```python
from build123d import *

# Parameters (mm, degrees)
SKETCH025_R     = 152.5
PAD015_DEPTH    = 8
SKETCH057_R     = 145.5
PAD016_DEPTH    = 4
SKETCH052_R     = 3
SKETCH052_R_2   = 1.5
SKETCH052_R_3   = 1
SKETCH052_R_4   = 2.75
POCKET018_DEPTH = 12.001


with BuildPart() as part:
    # Sketch025 → Pad015 (new body)
    with BuildSketch(Plane.XY):
        with Locations((0.142028, -323.737579)):
            Circle(SKETCH025_R)
    extrude(amount=PAD015_DEPTH)

    # Sketch057 (on DatumPlane) → Pad016 (join)
    with BuildSketch(Plane.XY.offset(8)):
        with Locations((0.142028, -323.737579)):
            Circle(SKETCH057_R)
    extrude(amount=PAD016_DEPTH)

    # Sketch052 → Pocket018 (cut, through all)
    with BuildSketch(Plane.XY.offset(12)):
        with Locations((0.142028, -183.237579)):
            Circle(SKETCH052_R)
        with Locations((133.765469, -280.320691)):
            Circle(SKETCH052_R)
        with Locations((110.940112, -287.737099)):
            Circle(SKETCH052_R_2)
        with Locations((-133.481413, -280.320691)):
            Circle(SKETCH052_R)
        with Locations((-110.656056, -287.737099)):
            Circle(SKETCH052_R_2)
        with Locations((-82.4418, -437.404467)):
            Circle(SKETCH052_R)
        with Locations((-68.334954, -417.988059)):
            Circle(SKETCH052_R_2)
        with Locations((82.725856, -437.404467)):
            Circle(SKETCH052_R)
        with Locations((68.61901, -417.988059)):
            Circle(SKETCH052_R_2)
        with Locations((-33.357972, -417.512577)):
            Circle(SKETCH052_R_3)
        with Locations((-33.357972, -457.512577)):
            Circle(SKETCH052_R_3)
        with Locations((33.642028, -457.512577)):
            Circle(SKETCH052_R_3)
        with Locations((33.642028, -417.512577)):
            Circle(SKETCH052_R_3)
        with Locations((0.142028, -207.237579)):
            Circle(SKETCH052_R_3)
        with Locations((-17.857972, -427.512577)):
            Circle(SKETCH052_R_4)
        with Locations((18.142028, -427.512577)):
            Circle(SKETCH052_R_4)
    extrude(amount=-POCKET018_DEPTH, mode=Mode.SUBTRACT)


with BuildPart() as part_1:
    # Body005 placement: moved
    add(part.part.moved(Location((154.819995, -19.410585, 0))))


solid = part_1.part
```
Source: CAD feature listing. Evaluate the final solid. Frame: model axes, mm. A direction names the side the tool comes from. Round coordinates to 2 decimals unless told otherwise and drop trailing zeros. Loops run counter-clockwise (first coordinate to the right, second up) from the corner with the lowest first, then second, coordinate; pieces in that order, holes last. Notation, with made-up numbers: M -4.5,-2.75 L 47.5,-2.75 A17 ccw 47.5,26.25 Z; hole C 45,32 d10. An arc over 180 degrees is marked long. Use a Markdown table: item, result. Add a question column.
1. Section query C-C on y = -250. Return the cut outline in (x, z).
2. Line query: line 1 (Y direction, x = 154.5, z = 5.25); line 2 (Y direction, x = 188, z = 6.5); line 3 (X direction, y = -307.5, z = 5). Output: solid intervals per line, ascending.
3. Section query A-A on z = 5.5. Give the number of separate pieces and of enclosed holes in the cut face, then the cut area to 3 significant figures.
4. Reachability of faces 1 (the cylindrical face through (9.6, -336.8, 10)), 2 (the flat face through (153, -341, 0)) from +Z, -Z, +X, -X, +Y, -Y: full face, straight path, thin tool, end or side. Return the list, or none.
5. Section query B-B on x = 161.5. Return the cut outline in (y, z).
6. Contact query for flat-ended pins moving along their axis: P1, Ø6, axis at y = -431.5, z = 3.5, coming from the +X side; P2, Ø3, axis at x = 223, z = 5.5, coming from the +Y side; P3, Ø1.5, axis at y = -446.5, z = 9.5, coming from the +X side. Output: stop coordinate, or through.
Reported:
| question | item | result |
|---|---|---|
| 1 | outline | M 34.22,0 L 275.71,0 L 275.71,8 L 266.74,8 L 266.74,12 L 43.19,12 L 43.19,8 L 34.22,8 Z |
| 2 | line 1 | y = -495.65 to -227.54, -225.76 to -205.61, -199.68 to -190.65 |
| 2 | line 2 | y = -492.03 to -477.81, -476.04 to -437.81, -436.04 to -194.27 |
| 2 | line 3 | x = 6.69 to 42.71, 45.62 to 264.3, 267.22 to 303.24 |
| 3 | separate pieces | 1 |
| 3 | enclosed holes | 16 |
| 3 | area | 72,800 mm² |
| 4 | face 1 | +Z |
| 4 | face 2 | -Z, +X, -X, +Y, -Y |
| 5 | outline | M -495.51,0 L -190.79,0 L -190.79,8 L -197.8,8 L -197.8,12 L -488.5,12 L -488.5,8 L -495.51,8 Z |
| 6 | P1 | stops at x = 281.34 |
| 6 | P2 | stops at y = -205.93 |
| 6 | P3 | stops at x = 258.13 |
